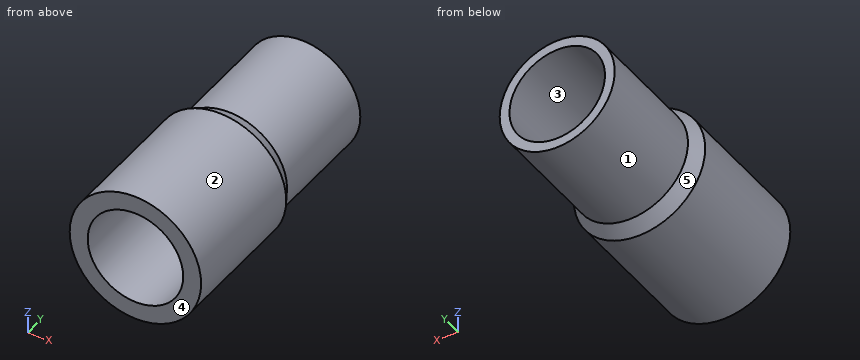
```python
from build123d import *

# Parameters (mm, degrees)
F0_R     = 50.8
F1_DEPTH = 203.2
F4_R     = 36.9189
F5_DEPTH = 203.2


with BuildPart() as f1:
    # F0 (on Front) → F1 (new body)
    with BuildSketch(Plane.XZ):
        Circle(F0_R)
    extrude(amount=F1_DEPTH)

    # F2 (on Top) → F3 (revolve, cut)
    with BuildSketch(Plane.XY):
        Polygon((89.635386, 0), (44.45, 0), (44.45, -88.9), (89.635386, -167.163385), align=None)
    revolve(axis=Axis((0, 0, 0), (0, 1, 0)), mode=Mode.SUBTRACT)

    # F4 (on face) → F5 (cut)
    with BuildSketch(Plane.XZ.offset(203.2)):
        Circle(F4_R)
    extrude(amount=-F5_DEPTH, mode=Mode.SUBTRACT)


solid = f1.part
```
Work out the finished part from the listing and answer in its coordinate system (mm). Face numbers are marked on the shaded views. A direction names the side the tool comes from. Round coordinates to 2 decimals unless told otherwise and drop trailing zeros. Loops run counter-clockwise (first coordinate to the right, second up) from the corner with the lowest first, then second, coordinate; pieces in that order, holes last. Notation, with made-up numbers: (14, 62) -> (29, 62) arc R25 ccw to (29, 101) -> close; hole circle Ø1 at (46, 70.5). An arc over 180 degrees is marked (long way). Write each question's results on one line, items separated by ' | '. Start each with the question number.
1. For a pull along Z with two mould halves and no side action, classify the marked faces 3, 4 and 5 as +Z half, -Z half, draft (parallel to the pull), parting line (faces both ways), or undercut.
2. Find the intervals of material crossed by probe 1 along Z at (x, y) = (0, -151); probe 2 along Z at (x, y) = (0, -84); probe 3 along X at (y, z) = (-60.5, -11), in increasing order. Write a range as from..to.
3. A tool of negligible diameter and unlimited length cuts with its end or side. For the marked faces 1 and 2, from which of +Z, -Z, +X, -X, +Y, -Y can it reach the whole face along a straight path? Write none if from no direction.
4. Section C-C (y = -45) is taken. Determine the outline of the cut face in (x, z).
5. Section D-D (y = -92) is taken. Determine the outline of the cut face in (x, z).
6. Section A-A (z = 0) is taken. Determine the outline of the cut face in (x, y).
7. Section B-B (x = 0) is taken. Determine the outline of the cut face in (y, z).
8. Given pin 1 Ø1.5 at (y, z) = (-62.5, 35.5) entering from +X; pin 2 Ø6 at (y, z) = (-21.5, -33) entering from -X; pin 3 Ø12 at (x, y) = (6.5, -125) entering from -Z; pin 4 Ø12 at (y, z) = (-145, -3.5) entering from -X, each flat-ended and moving along its own axis, determine where each tip first touches the part or whether it passes through.
Evaluation:
1) face 3: undercut | face 4: draft | face 5: parting line
2) probe 1: z = -50.8..-36.92, 36.92..50.8 | probe 2: z = -44.45..-36.92, 36.92..44.45 | probe 3: x = -43.07..-35.24, 35.24..43.07
3) face 1: +Y | face 2: +Y, -Y
4) outline: circle Ø88.9 at (0, 0); hole circle Ø73.84 at (0, 0)
5) outline: circle Ø92.48 at (0, 0); hole circle Ø73.84 at (0, 0)
6) outline: (-50.8, -203.2) -> (-36.92, -203.2) -> (-36.92, 0) -> (-44.45, 0) -> (-44.45, -88.9) -> (-50.8, -99.9) -> close; (36.92, -203.2) -> (50.8, -203.2) -> (50.8, -99.9) -> (44.45, -88.9) -> (44.45, 0) -> (36.92, 0) -> close
7) outline: (-203.2, -50.8) -> (-99.9, -50.8) -> (-88.9, -44.45) -> (0, -44.45) -> (0, -36.92) -> (-203.2, -36.92) -> close; (-203.2, 36.92) -> (0, 36.92) -> (0, 44.45) -> (-88.9, 44.45) -> (-99.9, 50.8) -> (-203.2, 50.8) -> close
8) pin 1: stops at x = 27.72 | pin 2: stops at x = -32.8 | pin 3: stops at z = -50.8 | pin 4: stops at x = -50.8
